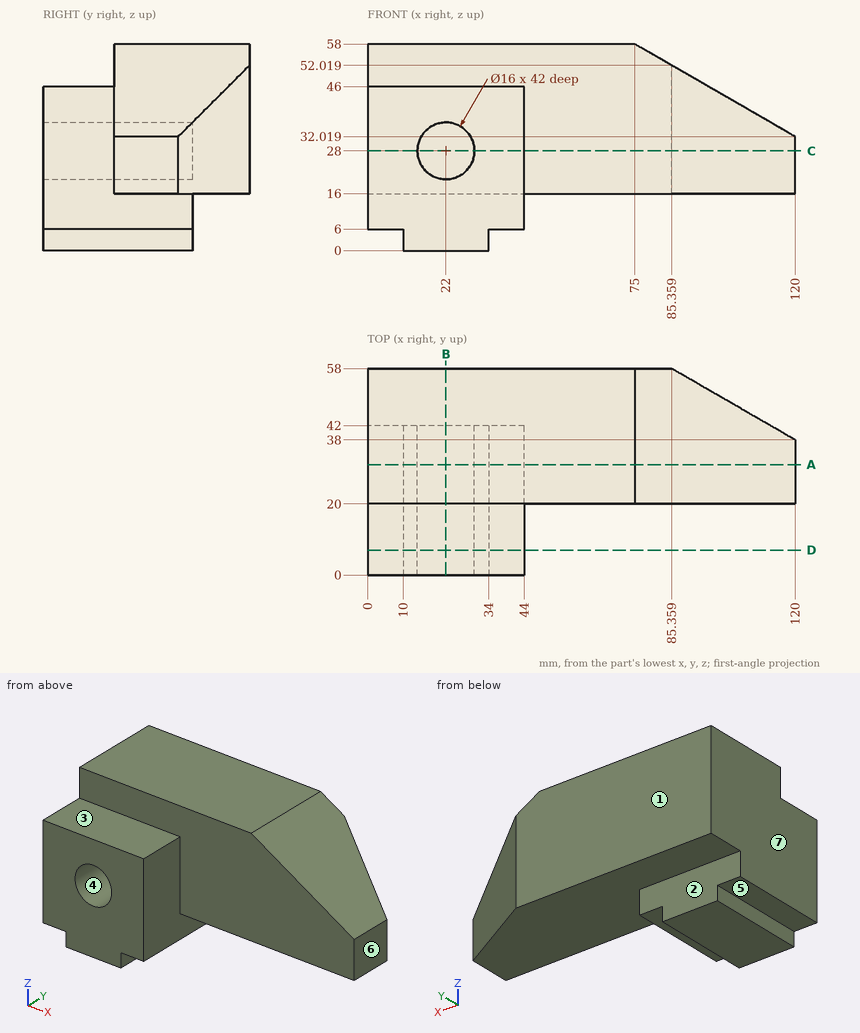
Geometry: see drawing. Coordinates: mm, zero at the bounding-box minimum. A direction names the side the tool comes from. Give positions to 0.01 mm unless a question says otherwise; leave off trailing zeros. Order: outer loops, then holes, each group sorted by start corner. A loop starts at its lowest first (then second) coordinate and runs counter-clockwise, first axis right, second up.
1. Cut plane D-D (y = 7). Return loops of the section in (x, z), and give its area (3 significant figures).
Computed:
outline: (0, 6) - (10, 6) - (10, 0) - (34, 0) - (34, 6) - (44, 6) - (44, 46) - (0, 46) - close; hole circle Ø16 at (22, 28)
area: 1,700 mm2
2. Line query: probe 1 along Z at (x, y) = (22, 11); probe 2 along Z at (x, y) = (22, 26); probe 3 along X at (y, z) = (31, 28). Output: solid intervals per line, ascending.
Computed:
probe 1: z = 0 to 20, 36 to 46
probe 2: z = 0 to 20, 36 to 58
probe 3: x = 0 to 14, 30 to 120
3. Set-up query: the marked faces 1, 2 and 3. Return all of +Z, -Z, +X, -X, +Y, -Y with unobstructed straight access to the full face (end or side cutting, diameter ignored); none if empty.
Computed:
face 1: +Z, -Z, +X, -X, +Y
face 2: -Z, +X, -X, +Y
face 3: +Z, +X, -X, -Y
4. Pin query (flat end, axial travel): pin 1 Ø12 at (x, y) = (25.5, 7) entering from +Z; pin 2 Ø12 at (x, y) = (86.5, 19) entering from +Z; pin 3 Ø8 at (x, z) = (21.5, 31.5) entering from -Y. Return the tip coordinate at first contact, or that it passes through.
Computed:
pin 1: stops at z = 46
pin 2: stops at z = 54.78
pin 3: stops at y = 42
5. Cut plane C-C (z = 28). Return loops of the section in (x, y).
Computed:
outline: (0, 0) - (14, 0) - (14, 42) - (30, 42) - (30, 0) - (44, 0) - (44, 20) - (120, 20) - (120, 38) - (85.36, 58) - (0, 58) - close
6. Cut plane B-B (x = 22). Return loops of the section in (y, z), and give its area (3 significant figures).
Computed:
outline: (0, 0) - (42, 0) - (42, 16) - (58, 16) - (58, 58) - (20, 58) - (20, 46) - (0, 46) - (0, 36) - (42, 36) - (42, 20) - (0, 20) - close
area: 2,200 mm2
7. Cut plane A-A (y = 31). Return loops of the section in (x, z), and give its area (3 significant figures).
Computed:
outline: (0, 6) - (10, 6) - (10, 0) - (34, 0) - (34, 6) - (44, 6) - (44, 16) - (120, 16) - (120, 32.02) - (75, 58) - (0, 58) - close; hole circle Ø16 at (22, 28)
area: 4,840 mm2
8. Draft query along X for the marked faces 4, 5, 6 and 7. Return one class per face: released by +X, released by -X, zero draft, split by the parting line, or undercut.
Computed:
face 4: undercut
face 5: zero draft
face 6: released by +X
face 7: released by -X
